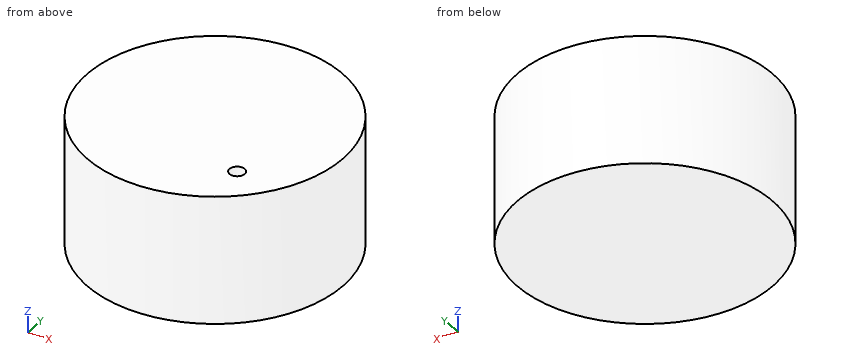
```python
from build123d import *

# Parameters (mm, degrees)
F0_R     = 50
F1_DEPTH = 25
F3_DEPTH = 25
F4_R     = 50
F4_R_2   = 3.0077087993
F5_DEPTH = 25


with BuildPart() as f1:
    # F0 (on Top) → F1 (new body)
    with BuildSketch(Plane.XY):
        Circle(F0_R)
    extrude(amount=F1_DEPTH)

    # F2 (on face) → F3 (join)
    with BuildSketch(Plane.XY.offset(25)):
        Polygon((-0.9346593793, 23.0941153177), (-20.4674202327, 10.7376188925), (-19.5327608534, -12.3564964252), (0.9346593793, -23.0941153177), (20.4674202327, -10.7376188925), (19.5327608534, 12.3564964252), align=None)
    extrude(amount=F3_DEPTH)

    # F4 (on face) → F5 (join)
    with BuildSketch(Plane.XY.offset(25)):
        Circle(F4_R)
        with Locations((24.0734647959, -25.4608131945)):
            Circle(F4_R_2, mode=Mode.SUBTRACT)
        Polygon((-0.9346593793, 23.0941153177), (19.5327608534, 12.3564964252), (20.4674202327, -10.7376188925), (0.9346593793, -23.0941153177), (-19.5327608534, -12.3564964252), (-20.4674202327, 10.7376188925), align=None, mode=Mode.SUBTRACT)
    extrude(amount=F5_DEPTH)


solid = f1.part
```
Part model, mm, in its own coordinate system. Round coordinates to 2 decimals unless told otherwise and drop trailing zeros. Write each loop counter-clockwise with the first axis right and the second up, starting at its lowest first coordinate (ties: lowest second). Pieces come first, ordered by that corner, then holes.
Item 1: Cut at B-B, the plane y = 30. Give the cut face in (x, z), plus the area to 3 significant figures.
Results:
outline: (-40, 0) - (40, 0) - (40, 50) - (-40, 50) - close
area: 4,000 mm2
Item 2: Drop flat-ended pins along their axis: pin 1 Ø10 at (y, z) = (-34, 37.5) entering from +X; pin 2 Ø8 at (x, z) = (37, 9) entering from -Y; pin 3 Ø3 at (x, z) = (26, 32.5) entering from -Y. Give the stop position or say it passes through.
Results:
pin 1: stops at x = 40.73
pin 2: stops at y = -37.56
pin 3: stops at y = -43.59
Item 3: Cut at C-C, the plane x = 35. Give the cut face in (y, z), plus the area to 3 significant figures.
Results:
outline: (-35.71, 0) - (35.71, 0) - (35.71, 50) - (-35.71, 50) - close
area: 3,570 mm2
Item 4: Probe L1, parallel to Y at x = 26, z = 31.5; L2, parallel to Y at x = -2, z = 6; L3, parallel to Y at x = 34, z = 9.5. List the from-to ranges inside material, lowest first.
Results:
L1: y = -42.71 to -27.77, -23.15 to 42.71
L2: y = -49.96 to 49.96
L3: y = -36.66 to 36.66
Item 5: Cut at D-D, the plane z = 31.5. Give the cut face in (x, y), plus the area to 3 significant figures.
Results:
outline: circle Ø100 at (0, 0); hole circle Ø6.02 at (24.07, -25.46)
area: 7,830 mm2
Item 6: Cut at A-A, the plane z = 6. Give the cut face in (x, y).
Results:
outline: circle Ø100 at (0, 0)
